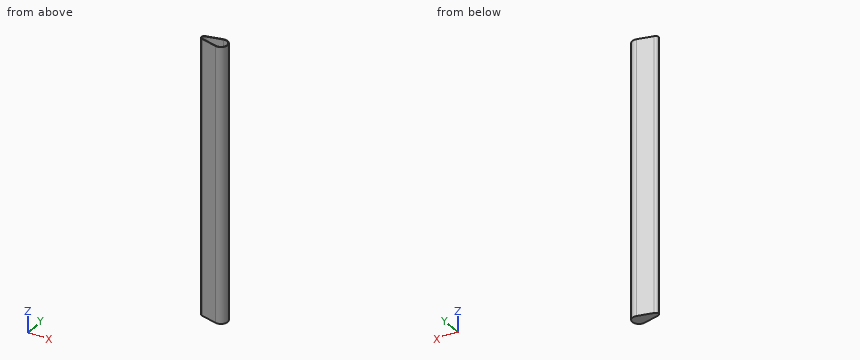
from build123d import *

# Parameters (mm, degrees)
F1_DEPTH = 1270
F2_T     = -2.54


with BuildPart() as f1:
    # F0 (on Top) → F1 (new body)
    with BuildSketch(Plane.XY):
        with BuildLine():
            Line((-76.2946611271, -13.1918803182), (-7.4450064273, -30.1775547845))
            ThreePointArc((-7.4450064273, -30.1775547845), (31.0823079854, -0.0553513609), (-7.3374791949, 30.2038794286))
            Line((-7.3374791949, 30.2038794286), (-77.4847210084, 13.1628920746))
            ThreePointArc((-77.4847210084, 13.1628920746), (-89.7500027986, -0.5952064431), (-76.2946611271, -13.1918803182))
        make_face()
    extrude(amount=F1_DEPTH)

    # F2
    f2_openings = [f1.faces().sort_by_distance(p)[0] for p in [
        (-22.239266, 0.032692, 1270),
    ]]
    offset(amount=F2_T, openings=f2_openings, kind=Kind.INTERSECTION)


solid = f1.part
The model under review builds one solid part; all positions refer to its coordinate system, in mm. Round coordinates to 2 decimals unless told otherwise and drop trailing zeros. Write each loop counter-clockwise with the first axis right and the second up, starting at its lowest first coordinate (ties: lowest second). Pieces come first, ordered by that corner, then holes. Notation, with made-up numbers: M -0.75,48.5 L 15.25,48.5 A17 cw 15.25,68.5 Z; hole C -25,53.5 d10. An arc over 180 degrees is marked long. Answer as CSV lines item,"result". Start each with the question number.
Q1. Consider section C-C, the plane x = 14. Give the boundary of the cut face in (y, z).
Q2. Clearance check with flat-ended pins moving along their axes: P1, Ø1, axis at x = -45, z = 188, coming from the +Y side; P2, Ø3, axis at x = -16, z = 681, coming from the +Y side; P3, Ø1.5, axis at x = -51.5, y = -21.5, coming from the +Z side; P4, Ø1, axis at y = -1.5, z = 273.5, coming from the -X side. State where each tip first meets the part, or that it passes through.
Q3. Consider section A-A, the plane z = 981. Give the boundary of the cut face in (x, y) (1 decimal), then the cut area to 3 significant figures.
Q4. Wall thickness on line 1 along Y through (x, z) = (0, 499.5); line 2 along Y through (x, z) = (-7.5, 610.5); line 3 along X through (y, z) = (0, 547): over which ranges is each line inside the solid? List them lowest first.
Q5. Consider section B-B, the plane y = 0. Give the boundary of the cut face in (x, z).
Result set:
1,outline,"M -27.75,0 L 27.75,0 L 27.75,1270 L 24.87,1270 L 24.87,2.54 L -24.87,2.54 L -24.87,1270 L -27.75,1270 Z"
2,P1,"stops at y = 21.18"
2,P2,"stops at y = 28.46"
2,P3,"passes through"
2,P4,"stops at x = -89.73"
3,outline,"M -77.5,13.2 A13.2 ccw -76.3,-13.2 L -7.4,-30.2 A31.1 ccw long -7.3,30.2 Z; hole M -77.1,10.6 A10.7 ccw -76,-10.6 L -6.8,-27.7 A28.5 ccw long -6.7,27.7 Z"
3,area,"733 mm²"
4,line 1,"y = -31.08 to -28.54, 28.54 to 31.08"
4,line 2,"y = -30.16 to -27.55, 27.55 to 30.16"
4,line 3,"x = -89.76 to -87.22, 28.54 to 31.08"
5,outline,"M -89.76,0 L 31.08,0 L 31.08,1270 L 28.54,1270 L 28.54,2.54 L -87.22,2.54 L -87.22,1270 L -89.76,1270 Z"
